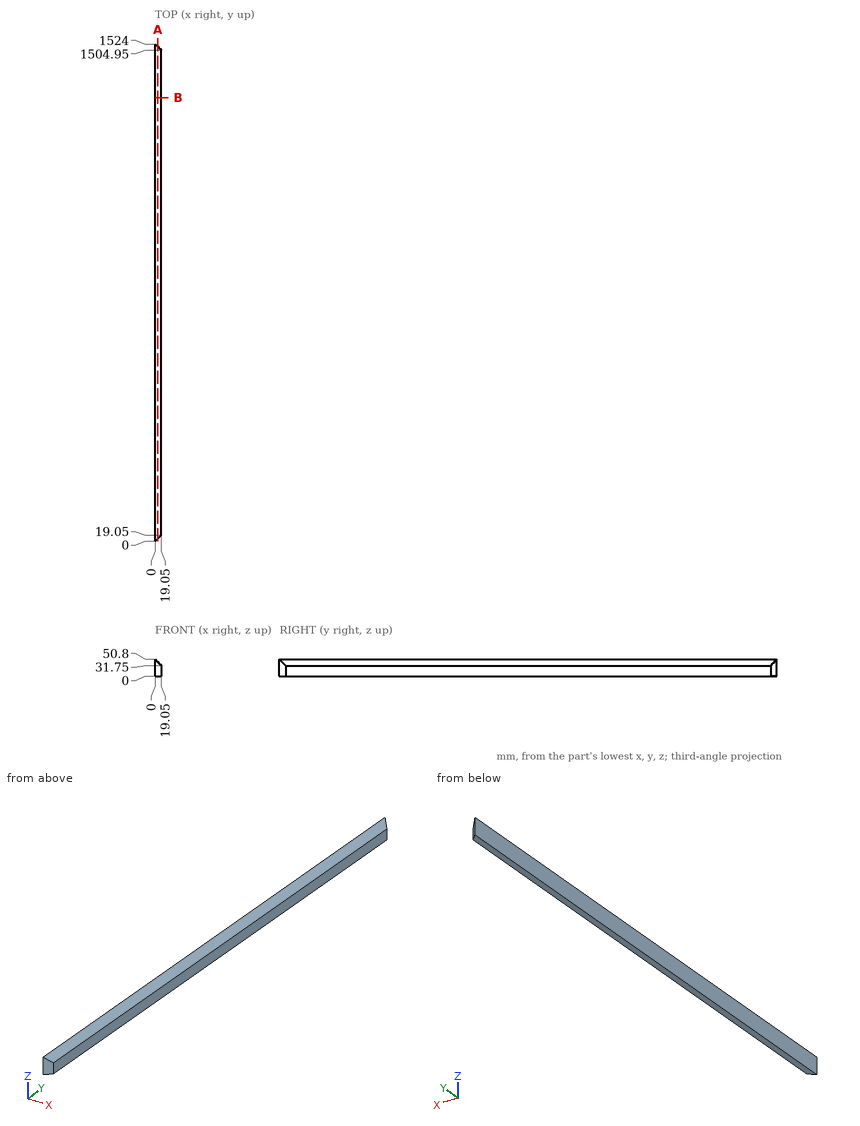
Part print with two shaded views. Sizes in mm from the minimum x, y, z corner. Coordinates: 2 decimals unless noted, no trailing zeros. Order: outer loops, then holes, each group sorted by start corner. A loop starts at its lowest first (then second) coordinate and runs counter-clockwise, first axis right, second up. Notation, with made-up numbers: (9.5, 73.5) - (37.5, 73.5) arc R35 cw to (37.5, 105.5) - close; hole circle Ø2 at (43, 27). An arc over 180 degrees is marked (long way). Write item = value, one per line. Start each with the question number.
1) Saw through at B-B on y = 1360. Write the cut outline in (x, z).
2) Saw through at A-A on x = 8.5. Write the cut outline in (y, z), then the cut area to 3 significant figures.
3) Flat gauge pins, fed straight in: pin 1 Ø8 at (y, z) = (1145.5, 39) entering from +X; pin 2 Ø5 at (x, y) = (5.5, 622) entering from +Z; pin 3 Ø2 at (x, z) = (8.5, 45) entering from +Y; pin 4 Ø6 at (x, y) = (7, 1364) entering from +Z. Where does each tip first touch, or does it go through?
4) Wall check: line 1 along X through (y, z) = (771, 44.5); line 2 along Y through (x, z) = (12, 26.5); line 3 along Z through (x, y) = (4.5, 1403). Give the ranges that are in metal, low to high. Write a range as from..to.
From the geometry:
q1.outline = (0, 0) - (19.05, 0) - (19.05, 31.75) - (0, 50.8) - close
q2.outline = (8.5, 0) - (1515.5, 0) - (1515.5, 42.3) - (8.5, 42.3) - close
q2.area = 63,700 mm^2
q3.pin_1 = 15.8
q3.pin_2 = 47.8
q3.pin_3 = through
q3.pin_4 = 46.8
q4.line_1 = 0..6.3
q4.line_2 = 12..1512
q4.line_3 = 0..46.3
